```python
from build123d import *

# Parameters (mm, degrees)
SALIENTE_EXTRUIR1_DEPTH = 1
SALIENTE_EXTRUIR2_DEPTH = 1


with BuildPart() as part:
    # Croquis1 → Saliente-Extruir1 (new body)
    with BuildSketch(Plane.XY):
        with BuildLine():
            Line((-102.798975089, 22.90959253), (-78.798975089, 22.90959253))
            ThreePointArc((-78.798975089, 22.90959253), (-69.298975089, 13.40959253), (-78.798975089, 3.90959253))
            Line((-78.798975089, 3.90959253), (-102.798975089, 3.90959253))
            ThreePointArc((-102.798975089, 3.90959253), (-112.298975089, 13.40959253), (-102.798975089, 22.90959253))
        make_face()
    extrude(amount=SALIENTE_EXTRUIR1_DEPTH)

    # Croquis2 → Saliente-Extruir2 (add)
    with BuildSketch(Plane.XY.offset(1)):
        Polygon((-90.798975089, 22.90959253), (-118.298975089, 22.90959253), (-118.298975089, 3.90959253), (-66.298975089, 3.90959253), (-66.298975089, 22.90959253), align=None)
    extrude(amount=SALIENTE_EXTRUIR2_DEPTH)


solid = part.part
```
Input: part model. Units: mm. Frame: model coordinates. A direction names the side the tool comes from. Coordinates: 2 decimals unless noted, no trailing zeros. Order: outer loops, then holes, each group sorted by start corner. A loop starts at its lowest first (then second) coordinate and runs counter-clockwise, first axis right, second up. Notation, with made-up numbers: (-10.75, 82.5) - (10.25, 82.5) arc R22 ccw to (10.25, 101.5) - close; hole circle Ø11 at (17, 45.5). An arc over 180 degrees is marked (long way). Put each result on its own line as item: value.
1. Cut plane B-B on x = -110. Return the cut outline in (y, z).
Report:
outline: (3.91, 1) - (7.21, 1) - (7.21, 0) - (19.61, 0) - (19.61, 1) - (22.91, 1) - (22.91, 2) - (3.91, 2) - close
2. Reachability of faces 1 (the face through (-68, 14, 1)), 2 (the face through (-112.297, 13.201, 0.493)), 3 (the face through (-93, 14, 2)) from +Z, -Z, +X, -X, +Y, -Y: full face, straight path, thin tool, end or side. Return the list, or none.
Report:
face 1: -Z, +X
face 2: -Z, -X
face 3: +Z, +X, -X, +Y, -Y
3. Cut plane A-A on y = 20. Return the cut outline in (x, z).
Report:
outline: (-118.3, 1) - (-109.64, 1) - (-109.64, 0) - (-71.96, 0) - (-71.96, 1) - (-66.3, 1) - (-66.3, 2) - (-118.3, 2) - close
4. Line query: line 1 along Z through (x, y) = (-115, 10.75); line 2 along X through (y, z) = (8.25, 0.55); line 3 along Y through (x, z) = (-74.5, 0.95). Output: solid intervals per line, ascending.
Report:
line 1: z = 1 to 2
line 2: x = -110.78 to -70.82
line 3: y = 4.94 to 21.88
5. Cut plane C-C on z = 0.7. Return the cut outline in (x, y).
Report:
outline: (-102.8, 3.91) - (-78.8, 3.91) arc R9.5 ccw to (-78.8, 22.91) - (-102.8, 22.91) arc R9.5 ccw to start
